Geometry: see drawing. Coordinates: mm, zero at the bounding-box minimum. A direction names the side the tool comes from. Round coordinates to 2 decimals unless told otherwise and drop trailing zeros. Loops run counter-clockwise (first coordinate to the right, second up) from the corner with the lowest first, then second, coordinate; pieces in that order, holes last. Notation, with made-up numbers: (57.5, -31) - (61.5, -31) arc R24 cw to (61.5, -4) - close; hole circle Ø3 at (20, -39). An arc over 180 degrees is marked (long way). Write item = value, one per line. Start each with the question number.
Item 1: Section A-A (z = 16). Return loops of the section in (x, y), plus the area to 3 significant figures.
Item 2: Section C-C (x = 29). Return loops of the section in (y, z).
Item 3: First-contact query: pin 1 (10 mm diameter, centred on x = 10, z = 25, fed in from -Y); pin 2 (4 mm diameter, centred on x = 16, z = 28, fed in from +Y); pin 3 (1.5 mm diameter, centred on x = 23.5, y = 4.5, fed in from +Z); pin 4 (4 mm diameter, centred on y = 7.5, z = 17.5, fed in from +X). Flat tips, straight axial feed; report the tip coordinate or a pass-through.
Item 4: Section D-D (y = 1.5). Return loops of the section in (x, z), plus the area to 3 significant figures.
Item 5: Line query: line 1 (X direction, y = 7, z = 16); line 2 (Y direction, x = 20, z = 6.5); line 3 (X direction, y = 9.25, z = 13). Output: solid intervals per line, ascending. Write a range as from..to.
Item 6: Access query for the marked faces 4 and 5. Directions: +Z, -Z, +X, -X, +Y, -Y. A direction counts if a zero-diameter tool reaches every point of the face in a straight line with its end or side. Return the directions, or none.
Item 7: Section B-B (x = 16). Return loops of the section in (y, z).
Item 8: Draft query along Z for the marked faces 1, 2 and 3. Return one class per face: pulls with the +Z half, pulls with the -Z half, needs draft (parallel to the pull), parting line crosses it, or undercut.
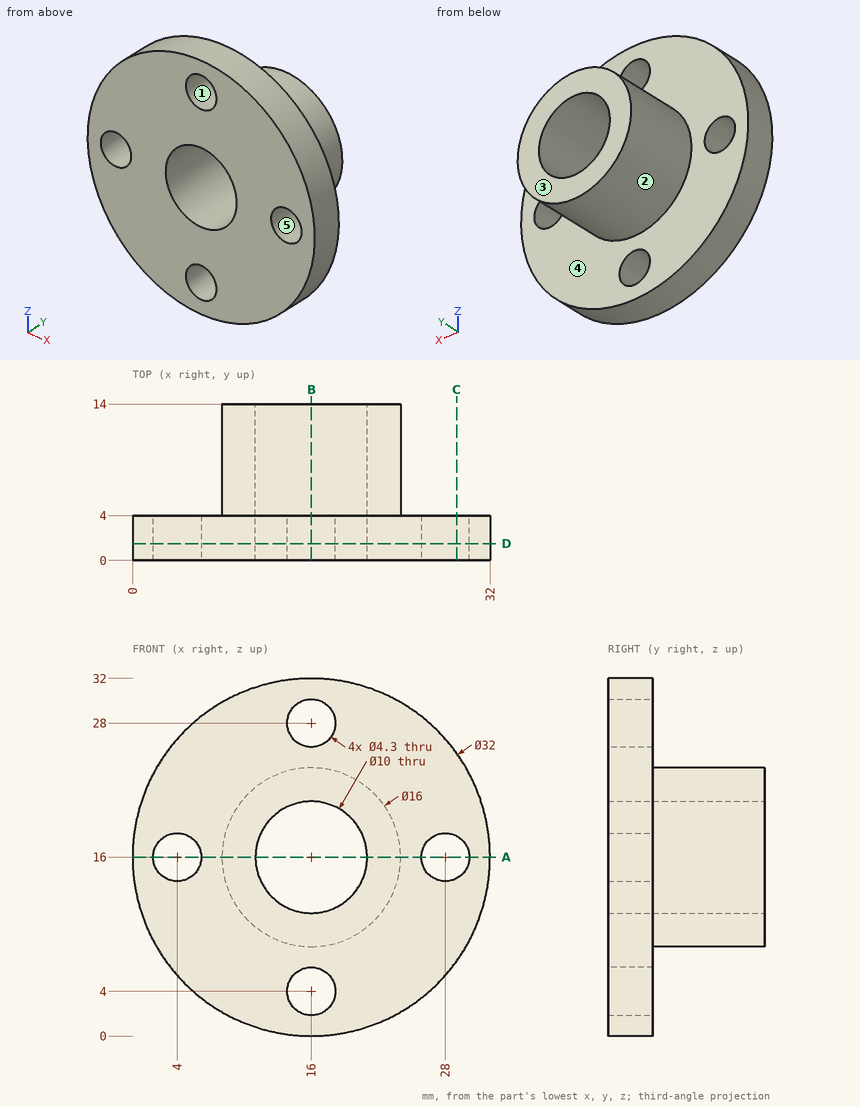
Taken from the geometry:
q1.outline = (0, 0) - (1.85, 0) - (1.85, 4) - (0, 4) - close; (6.15, 0) - (11, 0) - (11, 14) - (8, 14) - (8, 4) - (6.15, 4) - close; (21, 0) - (25.85, 0) - (25.85, 4) - (24, 4) - (24, 14) - (21, 14) - close; (30.15, 0) - (32, 0) - (32, 4) - (30.15, 4) - close
q1.area = 114 mm^2
q2.outline = (0, 6.67) - (4, 6.67) - (4, 14.1) - (0, 14.1) - close; (0, 17.9) - (4, 17.9) - (4, 25.33) - (0, 25.33) - close
q3.pin_1 = 0
q3.pin_2 = through
q3.pin_3 = 30.42
q3.pin_4 = 24
q4.outline = circle Ø32 at (16, 16); hole circle Ø4.3 at (4, 16); hole circle Ø10 at (16, 16); hole circle Ø4.3 at (16, 4); hole circle Ø4.3 at (16, 28); hole circle Ø4.3 at (28, 16)
q4.area = 668 mm^2
q5.line_1 = 8..11, 21..24
q5.line_2 = 0..4
q5.line_3 = 8.58..12, 20..23.42
q6.face_4 = +Y
q6.face_5 = +Y, -Y
q7.outline = (0, 0) - (4, 0) - (4, 1.85) - (0, 1.85) - close; (0, 6.15) - (4, 6.15) - (4, 8) - (14, 8) - (14, 11) - (0, 11) - close; (0, 21) - (14, 21) - (14, 24) - (4, 24) - (4, 25.85) - (0, 25.85) - close; (0, 30.15) - (4, 30.15) - (4, 32) - (0, 32) - close
q8.face_1 = undercut
q8.face_2 = parting line crosses it
q8.face_3 = needs draft
